Here's the drawing with two shaded views (mm, measured from the low corner). I have some questions. Give positions to 0.01 mm unless a question says otherwise; leave off trailing zeros. Loops run counter-clockwise (first coordinate to the right, second up) from the corner with the lowest first, then second, coordinate; pieces in that order, holes last. Notation, with made-up numbers: M 80,55.5 L 88,55.5 A37 cw 88,94.5 Z; hole C 35.5,-17.75 d1. An arc over 180 degrees is marked long. Use a Markdown table: item, result. Add a question column.
1) Suppose I cut it at C-C on z = 13.5. List the corners of the cut face in (x, y) for me, and give its area (3 significant figures).
2) Suppose I cut it at D-D on z = 22. List the corners of the cut face in (x, y) for me.
3) We'd pull the mould along X, two halves only. Please class the marked faces 1, 2 and 3: +X half, -X half, draft (parallel to the pull), parting line (faces both ways), or undercut.
4) Will these pins go through, and if not, where does the flat tip stop? pin 1 Ø4 at (x, z) = (4, 26.5) entering from -Y; pin 2 Ø1 at (y, z) = (11, 9) entering from +X; pin 3 Ø2 at (x, z) = (10, 35) entering from -Y.
5) Suppose I cut it at B-B on x = 8. List the corners of the cut face in (y, z) for me.
6) Suppose I cut it at A-A on y = 8. List the corners of the cut face in (x, z) for me.
7) If I drill on line 1 along X through (y, z) = (8.25, 22); line 2 along Z through (x, y) = (8, 5.25); line 3 along X through (y, z) = (9.25, 22), over which ranges is the centre line in solid material (lowest first)? Write a range as [from, to].
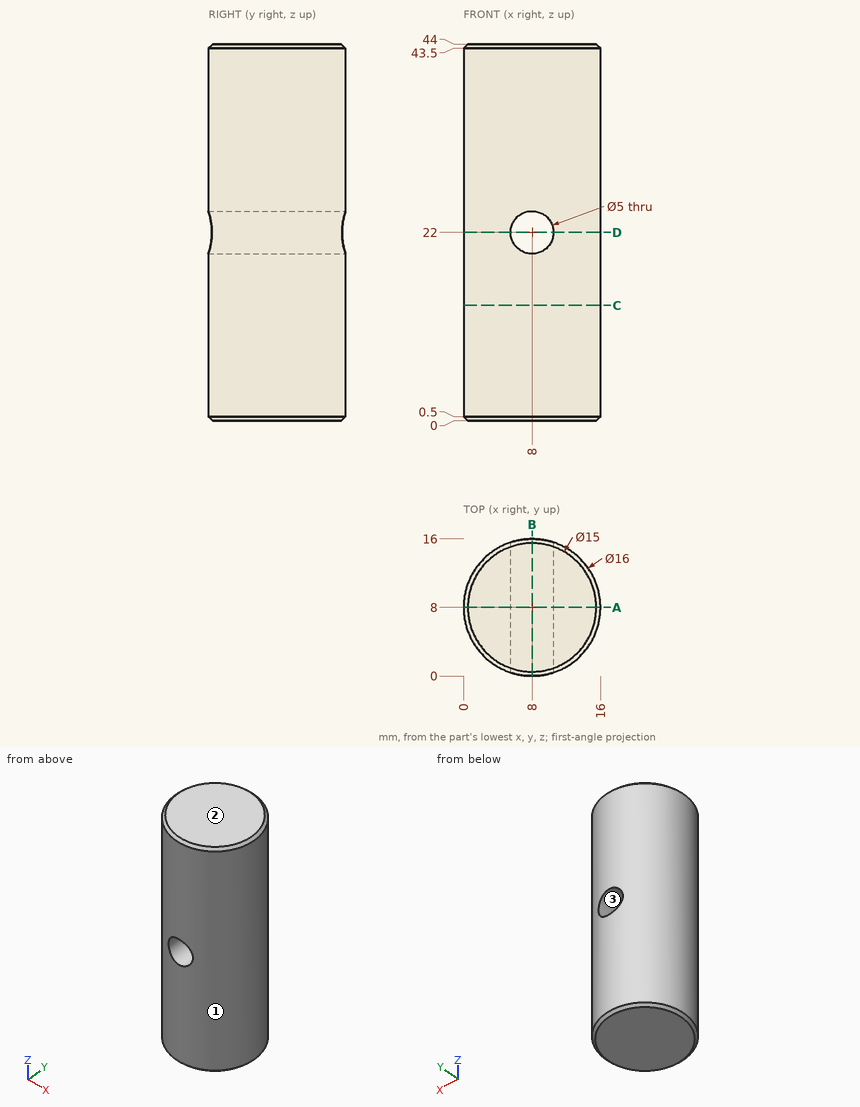
Answer block:
| question | item | result |
|---|---|---|
| 1 | outline | C 8,8 d16 |
| 1 | area | 201 mm^2 |
| 2 | outline | M 5.5,0.4 L 5.5,15.6 A8 ccw Z; M 10.5,0.4 A8 ccw 10.5,15.6 Z |
| 3 | face 1 | parting line |
| 3 | face 2 | draft |
| 3 | face 3 | undercut |
| 4 | pin 1 | stops at y = 0.25 |
| 4 | pin 2 | stops at x = 15.6 |
| 4 | pin 3 | stops at y = 0.06 |
| 5 | outline | M 0,0.5 L 0.5,0 L 15.5,0 L 16,0.5 L 16,19.5 L 0,19.5 Z; M 0,24.5 L 16,24.5 L 16,43.5 L 15.5,44 L 0.5,44 L 0,43.5 Z |
| 6 | outline | M 0,0.5 L 0.5,0 L 15.5,0 L 16,0.5 L 16,43.5 L 15.5,44 L 0.5,44 L 0,43.5 Z; hole C 8,22 d5 |
| 7 | line 1 | x = [0, 5.5], [10.5, 16] |
| 7 | line 2 | z = [0, 19.5], [24.5, 44] |
| 7 | line 3 | x = [0.1, 5.5], [10.5, 15.9] |
